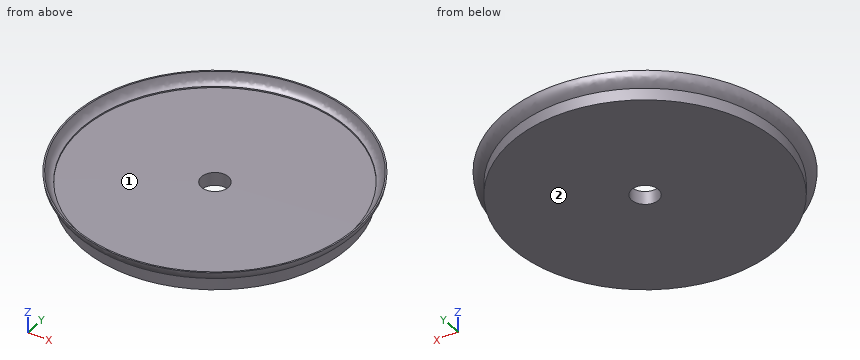
from build123d import *

# Parameters (mm, degrees)
SKETCH1_R           = 44.75
BOSS_EXTRUDE1_DEPTH = 4
SKETCH2_R           = 47.75
BOSS_EXTRUDE2_DEPTH = 4
SKETCH5_R           = 4.5
CUT_EXTRUDE1_DEPTH  = 10


with BuildPart() as part:
    # Sketch1 → Boss-Extrude1 (new body)
    with BuildSketch(Plane.XY):
        Circle(SKETCH1_R)
    extrude(amount=BOSS_EXTRUDE1_DEPTH)

    # Sketch2 → Boss-Extrude2 (add)
    with BuildSketch(Plane.XY.offset(4)):
        Circle(SKETCH2_R)
    extrude(amount=BOSS_EXTRUDE2_DEPTH)

    # Sketch3 → Cut-Revolve1 (revolve, cut)
    with BuildSketch(Plane(origin=(0, 0, 0), x_dir=(0, 0, -1), z_dir=(1, 0, 0))):
        with BuildLine():
            Line((-4, 47.75), (-4, 44.75))
            add(Edge.make_bspline(
                [(-4, 44.75), (-5.51655106, 47.70034682), (-8, 47.75)],
                knots=[0, 0, 0, 0.96689788, 0.96689788, 0.96689788], degree=2))
            Line((-8, 47.75), (-4, 47.75))
        make_face()
    revolve(axis=Axis((0, 0, 14.618090142), (0, 0, -1)), mode=Mode.SUBTRACT)

    # Sketch4 → Cut-Revolve3 (revolve, cut)
    with BuildSketch(Plane(origin=(0, 0, 0), x_dir=(0, 0, -1), z_dir=(1, 0, 0))):
        with BuildLine():
            Line((-4.667863656, 44.75), (-4.217612647, 44.75))
            Line((-4.217612647, 44.75), (-4.442738152, 0))
            Line((-4.442738152, 0), (-8, 0))
            Line((-8, 0), (-8, 47.272851402))
            add(Edge.make_bspline(
                [(-8, 47.272851402), (-5.020669257, 46.35865801), (-4.667863656, 44.75)],
                knots=[0, 0, 0, 0.52721511, 0.52721511, 0.52721511], degree=2))
        make_face()
    revolve(axis=Axis((0, 0, 4.442738152), (0, 0, 1)), mode=Mode.SUBTRACT)

    # Sketch5 → Cut-Extrude1 (cut)
    with BuildSketch(Plane(origin=(0, 0, 0), x_dir=(-1, 0, 0), z_dir=(0, 0, -1))):
        Circle(SKETCH5_R)
    extrude(amount=-CUT_EXTRUDE1_DEPTH, mode=Mode.SUBTRACT)


solid = part.part
Work out the finished part from the listing and answer in its coordinate system (mm). Face numbers are marked on the shaded views. Coordinates: 2 decimals unless noted, no trailing zeros. Write each loop counter-clockwise with the first axis right and the second up, starting at its lowest first coordinate (ties: lowest second). Pieces come first, ordered by that corner, then holes.
1. The part is cut by section A-A, the plane z = 1.25. Write down the section's boundary in (x, y).
Results list:
outline: circle Ø89.5 at (0, 0); hole circle Ø9 at (0, 0)
2. Flat-ended cylindrical pins translate along their axes: pin 1 (1.5 mm diameter, centred on x = -16.5, z = 1.5, fed in from +Y); pin 2 (1 mm diameter, centred on y = -19, z = 4, fed in from +X); pin 3 (7 mm diameter, centred on x = 0, y = 0, fed in from +Z); pin 4 (4 mm diameter, centred on x = -31, z = 2.5, fed in from -Y). Find the tip coordinate at first contact, or state that the pin passes through.
Results list:
pin 1: stops at y = 41.89
pin 2: stops at x = 41.49
pin 3: passes through
pin 4: stops at y = -34.08
3. Consider line 1 along X through (y, z) = (0, 2.65); line 2 along Z through (x, y) = (40, -11). Determine where each line is inside the solid, lowest interval first.
Results list:
line 1: x = -44.75 to -4.5, 4.5 to 44.75
line 2: z = 0 to 4.23
4. For a pull along X with two mould halves and no side action, classify the marked faces 1 and 2 as +X half, -X half, draft (parallel to the pull), parting line (faces both ways), or undercut.
Results list:
face 1: undercut
face 2: draft
